Build history of the part. All positions in model axes, mm. Face numbers are marked on the shaded views. Give positions to 0.01 mm unless a question says otherwise; leave off trailing zeros. Order: outer loops, then holes, each group sorted by start corner. A loop starts at its lowest first (then second) coordinate and runs counter-clockwise, first axis right, second up. Notation, with made-up numbers: (78, 73) -> (134, 73) arc R26 cw to (134, 95) -> close; hole circle Ø4 at (-23.5, -21.5). An arc over 180 degrees is marked (long way). One line per item, written item: value. Start each with the question number.
(1) Saw through at A-A on y = -27. Give the cut face in (x, z).
(2) Pin check, flat tips, straight feed: pin 1 (4 mm diameter, centred on y = 15.5, z = -7, fed in from -X); pin 2 (2 mm diameter, centred on y = 7, z = -5, fed in from -X); pin 3 (23 mm diameter, centred on x = 65, y = 0, fed in from +Z); pin 4 (1 mm diameter, centred on y = -10.5, z = -2, fed in from +X). Stop position of each tip, or through.
(3) Saw through at C-C on z = -6. Count the separate pieces of the cut face and the enclosed holes in it, plus the area to 3 significant figures.
(4) Saw through at B-B on x = 12. Give the cut face in (y, z), plus the area to 3 significant figures.
(5) Probe line 1 (Y direction, x = 0, z = -4.75); line 2 (X direction, y = 47.5, z = -8.5); line 3 (Y direction, x = 29, z = -4.5). List the from-to ranges inside material, lowest first.
(6) Two-plate mould, pull along Y, no slides. Class the marked faces 1, 2 and 3: +Y half, -Y half, draft (parallel to the pull), parting line (faces both ways), or undercut.
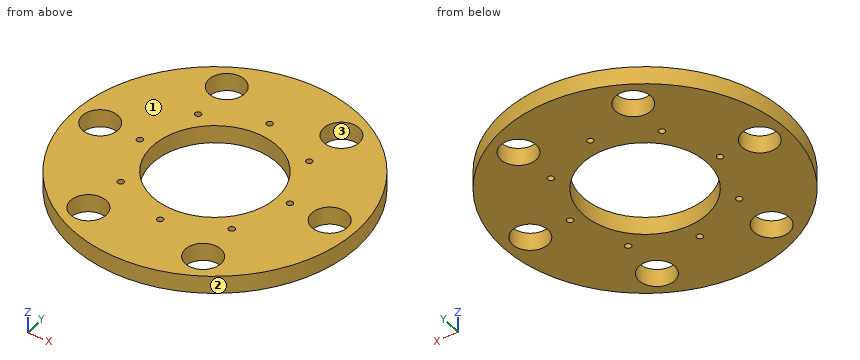
```python
from build123d import *

# Parameters (mm, degrees)
SKETCH_3_R          = 80
EXTRUDE_1_DEPTH     = 10
SKETCH_4_R          = 35
CUT_EXTRUDE_1_DEPTH = 7
SKETCH_6_R          = 10
CUT_EXTRUDE_3_DEPTH = 10
SKETCH_5_R          = 1.75
CUT_EXTRUDE_4_DEPTH = 10
SKETCH_7_R          = 35
CUT_EXTRUDE_5_DEPTH = 20


with BuildPart() as part:
    # 草图3 → 凸台-拉伸1 (new body)
    with BuildSketch(Plane.XY):
        Circle(SKETCH_3_R)
    extrude(amount=-EXTRUDE_1_DEPTH)

    # 草图4 → 切除-拉伸1 (cut)
    with BuildSketch(Plane.XY):
        Circle(SKETCH_4_R)
    extrude(amount=-CUT_EXTRUDE_1_DEPTH, mode=Mode.SUBTRACT)

    # 草图6 → 切除-拉伸3 (cut)
    with BuildSketch(Plane.XY):
        with Locations((-32.5, 56.291651246)):
            Circle(SKETCH_6_R)
        with BuildLine():
            ThreePointArc((-75, 0), (-65, -10), (-55, 0))
            Line((-55, 0), (-75, 0))
        make_face()
        with BuildLine():
            Line((-75, 0), (-55, 0))
            ThreePointArc((-55, 0), (-65, 10), (-75, 0))
        make_face()
        with Locations((-32.5, -56.291651246)):
            Circle(SKETCH_6_R)
        with Locations((32.5, -56.291651246)):
            Circle(SKETCH_6_R)
        with Locations((65, 0)):
            Circle(SKETCH_6_R)
        with Locations((32.5, 56.291651246)):
            Circle(SKETCH_6_R)
    extrude(amount=-CUT_EXTRUDE_3_DEPTH, mode=Mode.SUBTRACT)

    # 草图5 → 切除-拉伸4 (cut)
    with BuildSketch(Plane.XY):
        with Locations((0, 44.5)):
            Circle(SKETCH_5_R)
        with Locations((31.466251763, 31.466251763)):
            Circle(SKETCH_5_R)
        with Locations((42.5, 0)):
            Circle(SKETCH_5_R)
        with Locations((31.466251763, -31.466251763)):
            Circle(SKETCH_5_R)
        with Locations((-31.466251763, -31.466251763)):
            Circle(SKETCH_5_R)
        with BuildLine():
            ThreePointArc((-44.25, 0), (-42.5, -1.75), (-40.75, 0))
            Line((-40.75, 0), (-44.25, 0))
        make_face()
        with BuildLine():
            Line((-44.25, 0), (-40.75, 0))
            ThreePointArc((-40.75, 0), (-42.5, 1.75), (-44.25, 0))
        make_face()
        with Locations((-31.466251763, 31.466251763)):
            Circle(SKETCH_5_R)
        with Locations((0, -44.5)):
            Circle(SKETCH_5_R)
    extrude(amount=-CUT_EXTRUDE_4_DEPTH, mode=Mode.SUBTRACT)

    # 草图7 → 切除-拉伸5 (cut, symmetric)
    with BuildSketch(Plane.XY):
        Circle(SKETCH_7_R)
    extrude(amount=CUT_EXTRUDE_5_DEPTH, both=True, mode=Mode.SUBTRACT)


solid = part.part
```
Results below:
1. outline: (-75.31, -10) -> (-22.27, -10) -> (-22.27, 0) -> (-75.31, 0) -> close; (22.27, -10) -> (75.31, -10) -> (75.31, 0) -> (22.27, 0) -> close
2. pin 1: stops at x = -78.85
2. pin 2: stops at x = -79.77
2. pin 3: stops at z = 0
2. pin 4: stops at x = 79.37
3. separate pieces: 1
3. enclosed holes: 15
3. area: 14,300 mm²
4. outline: (-79.09, -10) -> (-32.88, -10) -> (-32.88, 0) -> (-79.09, 0) -> close; (32.88, -10) -> (79.09, -10) -> (79.09, 0) -> (32.88, 0) -> close
4. area: 924 mm²
5. line 1: y = -80 to -46.25, -42.75 to -35, 35 to 42.75, 46.25 to 80
5. line 2: x = -64.37 to -37.27, -27.73 to 27.73, 37.27 to 64.37
5. line 3: y = -74.56 to -65.66, -46.92 to -19.6, 19.6 to 46.92, 65.66 to 74.56
6. face 1: draft
6. face 2: parting line
6. face 3: undercut
